```python
from build123d import *

# Parameters (mm, degrees)
SKETCH1_W           = 38.101827682
SKETCH1_H           = 38.101827682
BOSS_EXTRUDE1_DEPTH = 25.4
CUT_EXTRUDE1_DEPTH  = 13.4
SKETCH4_R           = 8.523044684
CUT_EXTRUDE2_DEPTH  = 12


with BuildPart() as part:
    # Sketch1 → Boss-Extrude1 (new body)
    with BuildSketch(Plane(origin=(0, 0, 0), x_dir=(1, 0, 0), z_dir=(0, 1, 0))):
        with Locations((19.050913841, 19.050913841)):
            Rectangle(SKETCH1_W, SKETCH1_H)
    extrude(amount=BOSS_EXTRUDE1_DEPTH)

    # Sketch2 → Cut-Extrude1 (cut)
    with BuildSketch(Plane(origin=(0, 25.4, 0), x_dir=(1, 0, 0), z_dir=(0, 1, 0))):
        Polygon((33.100912857, 19.050913841), (26.075913349, 31.218569912), (12.025914333, 31.218569912), (5.000914826, 19.050913841), (12.025914333, 6.883257771), (26.075913349, 6.883257771), align=None)
    extrude(amount=-CUT_EXTRUDE1_DEPTH, mode=Mode.SUBTRACT)

    # Sketch4 → Cut-Extrude2 (cut)
    with BuildSketch(Plane.XZ):
        with Locations((19.050913841, -19.050913841)):
            Circle(SKETCH4_R)
    extrude(amount=-CUT_EXTRUDE2_DEPTH, mode=Mode.SUBTRACT)


solid = part.part
```
Geometry: final body of the model. Coordinates: model frame, mm. A direction names the side the tool comes from. Coordinates: 2 decimals unless noted, no trailing zeros. Order: outer loops, then holes, each group sorted by start corner. A loop starts at its lowest first (then second) coordinate and runs counter-clockwise, first axis right, second up. Notation, with made-up numbers: (-11, 56) - (48, 56) arc R19 cw to (48, 83) - close; hole circle Ø3 at (-23, 5.5). An arc over 180 degrees is marked (long way). Write each question's results on one line, items separated by ' | '.
1) Pin query (flat end, axial travel): pin 1 (12 mm diameter, centred on x = 13, z = -18.5, fed in from +Y). Return the tip coordinate at first contact, or that it passes through.
Results list:
pin 1: y = 12
2) Pull-direction query (X, two-part tool) for faces 1 (the flat face through (0, 13, -19)), 2 (the cylindrical face through (12.29, 5.92, -24.24)), 3 (the flat face through (19, 13, -38.102)); classes: pulls with the +X half, pulls with the -X half, needs draft (parallel to the pull), parting line crosses it, or undercut.
Results list:
face 1: pulls with the -X half | face 2: undercut | face 3: needs draft
3) Set-up query: faces 4 (the flat face through (19, 19, -6.883)), 5 (the flat face through (10, 0, -19)). Return all of +Z, -Z, +X, -X, +Y, -Y with unobstructed straight access to the full face (end or side cutting, diameter ignored); none if empty.
Results list:
face 4: +Y | face 5: +Z, -Z, +X, -X, -Y
4) Section D-D, the plane x = 10. Return loops of the section in (y, z), plus the area to 3 significant figures.
Results list:
outline: (0, -38.1) - (25.4, -38.1) - (25.4, -27.71) - (12, -27.71) - (12, -10.39) - (25.4, -10.39) - (25.4, 0) - (0, 0) - close | area: 736 mm^2
5) Section C-C, the plane z = -13. Return loops of the section in (x, y), plus the area to 3 significant figures.
Results list:
outline: (0, 0) - (13.05, 0) - (13.05, 12) - (8.49, 12) - (8.49, 25.4) - (0, 25.4) - close; (25.05, 0) - (38.1, 0) - (38.1, 25.4) - (29.61, 25.4) - (29.61, 12) - (25.05, 12) - close | area: 541 mm^2
6) Section B-B, the plane x = 20. Return loops of the section in (y, z), plus the area to 3 significant figures.
Results list:
outline: (0, -38.1) - (25.4, -38.1) - (25.4, -31.22) - (12, -31.22) - (12, -27.52) - (0, -27.52) - close; (0, -10.58) - (12, -10.58) - (12, -6.88) - (25.4, -6.88) - (25.4, 0) - (0, 0) - close | area: 438 mm^2
7) Line query: line 1 (Z direction, x = 23.5, y = 20.25); line 2 (Y direction, x = 15, z = -30); line 3 (X direction, y = 7.75, z = -13). Output: solid intervals per line, ascending. Write a range as from..to.
Results list:
line 1: -38.1..-31.22, -6.88..0 | line 2: 0..12 | line 3: 0..13.05, 25.05..38.1
8) Section A-A, the plane y = 23.5. Return loops of the section in (x, z).
Results list:
outline: (0, -38.1) - (38.1, -38.1) - (38.1, 0) - (0, 0) - close; hole (5, -19.05) - (12.03, -31.22) - (26.08, -31.22) - (33.1, -19.05) - (26.08, -6.88) - (12.03, -6.88) - close
